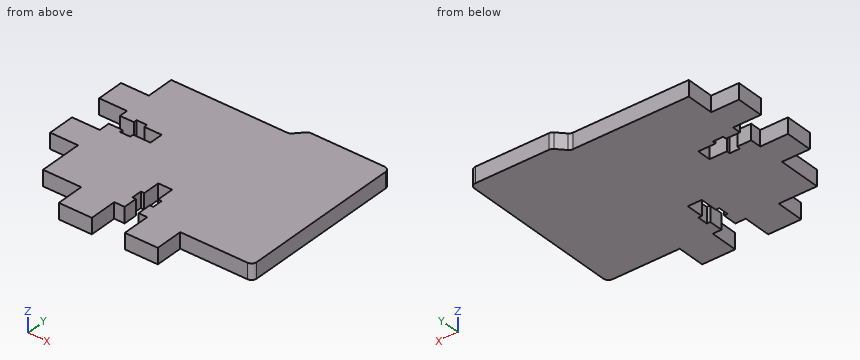
from build123d import *

# Parameters (mm, degrees)
F1_DEPTH = 4.5


with BuildPart() as f1:
    # F0 (on Top) → F1 (new body)
    with BuildSketch(Plane.XY):
        with BuildLine():
            Line((13.791552, 28.438764), (-19.5586, 28.438764))
            Line((-19.5586, 28.438764), (-19.5586, 20.438764))
            Line((-19.5586, 20.438764), (-27.5586, 20.438764))
            Line((-27.5586, 20.438764), (-27.5586, 12.638764))
            Line((-27.5586, 12.638764), (-19.5586, 12.638764))
            Line((-19.5586, 12.638764), (-19.5586, 10.138764))
            Line((-19.5586, 10.138764), (-15.5586, 10.138764))
            Line((-15.5586, 10.138764), (-15.5586, 11.138764))
            Line((-15.5586, 11.138764), (-12.5586, 11.138764))
            Line((-12.5586, 11.138764), (-12.5586, 10.138764))
            Line((-12.5586, 10.138764), (-7.5586, 10.138764))
            Line((-7.5586, 10.138764), (-7.5586, 6.138764))
            Line((-7.5586, 6.138764), (-12.5586, 6.138764))
            Line((-12.5586, 6.138764), (-12.5586, 5.138764))
            Line((-12.5586, 5.138764), (-15.5586, 5.138764))
            Line((-15.5586, 5.138764), (-15.5586, 6.138764))
            Line((-15.5586, 6.138764), (-19.5586, 6.138764))
            Line((-19.5586, 6.138764), (-19.5586, 2.938764))
            Line((-19.5586, 2.938764), (-27.5586, 2.938764))
            Line((-27.5586, 2.938764), (-27.5586, -4.861236))
            Line((-27.5586, -4.861236), (-19.5586, -4.861236))
            Line((-19.5586, -4.861236), (-19.5586, -12.361236))
            Line((-19.5586, -12.361236), (-19.5586, -17.361236))
            Line((-19.5586, -17.361236), (-11.749149, -17.361236))
            Line((-11.749149, -17.361236), (-8.5586, -17.361236))
            Line((-8.5586, -17.361236), (-8.5586, -25.361236))
            Line((-8.5586, -25.361236), (0.9414, -25.361236))
            Line((0.9414, -25.361236), (0.9414, -17.361236))
            Line((0.9414, -17.361236), (3.9414, -17.361236))
            Line((3.9414, -17.361236), (3.9414, -13.361236))
            Line((3.9414, -13.361236), (2.9414, -13.361236))
            Line((2.9414, -13.361236), (2.9414, -10.361236))
            Line((2.9414, -10.361236), (3.9414, -10.361236))
            Line((3.9414, -10.361236), (3.9414, -5.361236))
            Line((3.9414, -5.361236), (7.9414, -5.361236))
            Line((7.9414, -5.361236), (7.9414, -10.361236))
            Line((7.9414, -10.361236), (8.9414, -10.361236))
            Line((8.9414, -10.361236), (8.9414, -13.361236))
            Line((8.9414, -13.361236), (7.9414, -13.361236))
            Line((7.9414, -13.361236), (7.9414, -17.361236))
            Line((7.9414, -17.361236), (10.4414, -17.361236))
            Line((10.4414, -17.361236), (10.4414, -25.361236))
            Line((10.4414, -25.361236), (19.9414, -25.361236))
            Line((19.9414, -25.361236), (19.9414, -17.361236))
            Line((19.9414, -17.361236), (39.250851, -17.361236))
            ThreePointArc((39.250851, -17.361236), (40.311511, -16.921896), (40.750851, -15.861236))
            Line((40.750851, -15.861236), (40.750851, 30.138764))
            ThreePointArc((40.750851, 30.138764), (40.311511, 31.199425), (39.250851, 31.638764))
            Line((39.250851, 31.638764), (18.091248, 31.638764))
            ThreePointArc((18.091248, 31.638764), (17.494954, 31.515149), (16.996942, 31.164676))
            Line((16.996942, 31.164676), (14.885857, 28.912853))
            ThreePointArc((14.885857, 28.912853), (14.387845, 28.56238), (13.791552, 28.438764))
        make_face()
    extrude(amount=F1_DEPTH)


solid = f1.part
Input: part model. Units: mm. Frame: model coordinates. Give positions to 0.01 mm unless a question says otherwise; leave off trailing zeros. Order: outer loops, then holes, each group sorted by start corner. A loop starts at its lowest first (then second) coordinate and runs counter-clockwise, first axis right, second up. Notation, with made-up numbers: (-18, 39.5) - (-12, 39.5) arc R23 ccw to (-12, 78.5) - close; hole circle Ø1 at (15, -15). An arc over 180 degrees is marked (long way). Answer as a JSON object with one key per item and string values. Group by question number.
Q1. Cut plane A-A, the plane y = -19. Output: boundary loops of the cut face in (x, z), then the cut area to 3 significant figures.
Q2. Cut plane D-D, the plane x = -1. Output: boundary loops of the cut face in (y, z).
Q3. Line query: probe 1 along Y at (x, z) = (-12, 4.05); probe 2 along X at (y, z) = (-13, 3.9); probe 3 along Y at (x, z) = (8, 3.1). Output: solid intervals per line, ascending.
Q4. Cut plane B-B, the plane x = -21.5. Output: boundary loops of the cut face in (y, z), then the cut area to 3 significant figures.
Q5. Cut plane C-C, the plane y = 8.5. Output: boundary loops of the cut face in (x, z), then the cut area to 3 significant figures.
Q6. First-contact query: pin 1 Ø1.6 at (y, z) = (4.5, 2.5) entering from -X; pin 2 Ø2 at (x, z) = (-17, 2) entering from -Y; pin 3 Ø0.9 at (x, z) = (-13.5, 1) entering from +Y. Flat tips, straight axial feed; report the tip coordinate or a pass-through.
Results:
{
 "1": {"outline": "(-8.56, 0) - (0.94, 0) - (0.94, 4.5) - (-8.56, 4.5) - close; (10.44, 0) - (19.94, 0) - (19.94, 4.5) - (10.44, 4.5) - close", "area": "85.5 mm^2"},
 "2": {"outline": "(-25.36, 0) - (28.44, 0) - (28.44, 4.5) - (-25.36, 4.5) - close"},
 "3": {"probe 1": "-17.36 to 6.14, 10.14 to 28.44", "probe 2": "-19.56 to 2.94, 8.94 to 40.75", "probe 3": "-17.36 to -13.36, -10.36 to 28.44"},
 "4": {"outline": "(-4.86, 0) - (2.94, 0) - (2.94, 4.5) - (-4.86, 4.5) - close; (12.64, 0) - (20.44, 0) - (20.44, 4.5) - (12.64, 4.5) - close", "area": "70.2 mm^2"},
 "5": {"outline": "(-7.56, 0) - (40.75, 0) - (40.75, 4.5) - (-7.56, 4.5) - close", "area": "217 mm^2"},
 "6": {"pin 1": "x = -19.56", "pin 2": "y = -17.36", "pin 3": "y = 28.44"}
}
